Read the model definition and answer for the solid it produces. Units are mm, in the model's axes. Give positions to 0.01 mm unless a question says otherwise; leave off trailing zeros. Loops run counter-clockwise (first coordinate to the right, second up) from the corner with the lowest first, then second, coordinate; pieces in that order, holes last. Notation, with made-up numbers: (33, 61) - (44, 61) arc R22 cw to (44, 92) - close; hole circle Ø1 at (83.5, 62.25). An arc over 180 degrees is marked (long way). Put each result on its own line as item: value. Start each with the question number.
1. Given pin 1 Ø1.4 at (x, z) = (-68.66, 39.64) entering from -Y; pin 2 Ø8 at (x, z) = (7.5, 42) entering from -Y; pin 3 Ø1.5 at (x, z) = (-38, 49.5) entering from -Y; pin 4 Ø1.5 at (x, z) = (15, -41.5) entering from +Y, each flat-ended and moving along its own axis, determine where each tip first touches the part or whether it passes through.
2. For a pull along Z with two mould halves and no side action, classify faces 1 (the flat face through (24, 3.175, 73)), 2 (the cylindrical face through (-76.08, 1.57, 31.54)), 3 (the cylindrical face through (1.38, 31.26, 6.2)) as released by +Z, released by -Z, zero draft, split by the parting line, or undercut.
3. Consider L1, parallel to X at y = 4, z = 23.5; L2, parallel to Z at x = -30, y = 10.5; L3, parallel to X at y = 13.5, z = 31.5. Determine where each line is inside the solid, lowest interval first. Write a range as from..to.
4. A cutting plane is placed at A-A, the plane y = 25. Determine the outline of the cut face in (x, z).
```python
from build123d import *

# Parameters (mm, degrees)
CSK_FOR_0_FLAT_HEAD_MACHINE_SCREW_100_D           = 1.778
CSK_FOR_0_FLAT_HEAD_MACHINE_SCREW_100_CSINK_D     = 3.0226
CSK_FOR_0_FLAT_HEAD_MACHINE_SCREW_100_CSINK_ANGLE = 100
CIRPATTERN1_COUNT                                 = 12


with BuildPart() as part:
    # Sketch1 → Revolve1 (revolve)
    with BuildSketch(Plane.XY):
        with BuildLine():
            Line((-82.3595, 0), (-76.2, 0))
            ThreePointArc((-76.2, 0), (-75.836445405, 1.67032541), (-74.811557259, 3.038449384))
            ThreePointArc((-74.811557259, 3.038449384), (-42.880368086, 22.574179563), (-6.35, 30.745948226))
            Line((-6.35, 30.745948226), (-6.35, 31.763505888))
            ThreePointArc((-6.35, 31.763505888), (-43.680101788, 23.345613205), (-76.2, 3.175))
            Line((-76.2, 3.175), (-82.3595, 3.175))
            Line((-82.3595, 3.175), (-82.3595, 0))
        make_face()
    revolve(axis=Axis((0, 55, 0), (0, -1, 0)))

    # CSK for #0 Flat Head Machine Screw (100)1 (through all)
    with Locations(Plane(origin=(0, 3.175, 0), x_dir=(1, 0, 0), z_dir=(0, 1, 0))):
        with Locations((-79.27975, 0)):
            csk_for_0_flat_head_machine_screw_100 = CounterSinkHole(CSK_FOR_0_FLAT_HEAD_MACHINE_SCREW_100_D / 2, CSK_FOR_0_FLAT_HEAD_MACHINE_SCREW_100_CSINK_D / 2, counter_sink_angle=CSK_FOR_0_FLAT_HEAD_MACHINE_SCREW_100_CSINK_ANGLE)

    # CirPattern1: CSK for #0 Flat Head Machine Screw (100)1 ×12 about axis
    cirpattern1_axis = Axis((0, 0, 0), (0, 1, 0))
    for i in range(1, CIRPATTERN1_COUNT):
        add(csk_for_0_flat_head_machine_screw_100.rotate(cirpattern1_axis, i * 360 / CIRPATTERN1_COUNT), mode=Mode.SUBTRACT)


solid = part.part
```
Return value:
1. pin 1: passes through
1. pin 2: stops at y = 20.96
1. pin 3: stops at y = 11.89
1. pin 4: stops at y = 23.47
2. face 1: zero draft
2. face 2: split by the parting line
2. face 3: undercut
3. L1: x = -71.49..-69.84, 69.84..71.49
3. L2: z = -59.87..-57.89, 57.89..59.87
3. L3: x = -54.04..-51.84, 51.84..54.04
4. outline: circle Ø78.79 at (0, 0); hole circle Ø72.63 at (0, 0)
